Source: CAD feature listing. Evaluate the final solid. Frame: model axes, mm. A direction names the side the tool comes from. Give positions to 0.01 mm unless a question says otherwise; leave off trailing zeros. Loops run counter-clockwise (first coordinate to the right, second up) from the corner with the lowest first, then second, coordinate; pieces in that order, holes last.
Autodesk Inventor part; units mm, degrees
ref_plane "YZ Plane" through (0, 0, 0) normal (1, 0, 0) x (0, 1, 0)
ref_plane "XZ Plane" through (0, 0, 0) normal (0, 1, 0) x (-1, 0, 0)
ref_plane "XY Plane" through (0, 0, 0) normal (0, 0, 1) x (1, 0, 0)
sketch "Sketch1" plane through (0, 0, 0) normal (0, 1, 0) x (-1, 0, 0)
  line L0 (0, 0) -> (21.7678, 0)
  line L1 (21.7678, 0) -> (21.7678, -12.7)
  line L2 (21.7678, -12.7) -> (0, -12.7)
  line L3 (0, -12.7) -> (0, 0)
  circle A0 centre (25.7678, -10.95) radius 1.75
  circle A1 centre (-4, -1.75) radius 1.75
  circle A2 centre (25.7678, -10.95) radius 2.75
  circle A3 centre (-4, -1.75) radius 2.75
  line L4 (-1, -13.7) -> (22.7678, -13.7)
  line L5 (22.7678, -13.7) -> (22.7678, 1)
  line L6 (22.7678, 1) -> (-1, 1)
  line L7 (-1, 1) -> (-1, -13.7)
  line L8 (25.7678, -13.7) -> (22.7678, -13.7)
  line L9 (25.7678, -8.2) -> (22.7678, -8.2)
  line L10 (-4, 1) -> (-1, 1)
  line L11 (-4, -4.5) -> (-1, -4.5)
  dimension "d0" = 21.7678
  dimension "d1" = 12.7
  dimension "d2" = 3.5
  dimension "d3" = 3.5
  dimension "d4" = 4
  dimension "d5" = 4
  dimension "d6" = 5.5
  dimension "d7" = 5.5
extrude "Extrusion1" add sketch "Sketch1" along normal blind 2 contours L0 L1 L2 L3 | A2 | A2 L8 L5 L9 | L5 L4 L7 L6 | L7 L11 A3 L10 | A3
equation "\"d3\" = d2"
equation "\"d5\" = d4"
equation "\"d7\" = d6"
properties part number "HDMI Mount"
(1) Reachability of faces 1 (the flat face through (-22.768, 1, -4)), 2 (the flat face through (1, 1, -9)), 3 (the cylindrical face through (-24.02, 0.99, -11.03)) from +Z, -Z, +X, -X, +Y, -Y: full face, straight path, thin tool, end or side. Return the list, or none.
A:
face 1: +Z, -X, +Y, -Y
face 2: -Z, +X, +Y, -Y
face 3: +Y, -Y
(2) Section A-A, the plane y = 0.7. Return the cut outline in (x, z), then the cut area to 3 significant figures.
A:
outline: (-25.77, -13.7) - (1, -13.7) - (1, -4.5) - (4, -4.5) arc R2.75 ccw to (4, 1) - (-22.77, 1) - (-22.77, -8.2) - (-25.77, -8.2) arc R2.75 ccw to start; hole circle Ø3.5 at (-25.77, -10.95); hole circle Ø3.5 at (4, -1.75)
area: 387 mm2
(3) First-contact query: pin 1 (1 mm diameter, centred on y = 1, z = -9, fed in from -X); pin 2 (0.6 mm diameter, centred on y = 1, z = -10.5, fed in from +X). Flat tips, straight axial feed; report the tip coordinate or a pass-through.
A:
pin 1: stops at x = -28.1
pin 2: stops at x = 1
(4) Ray query, line 1 along Z through (x, y) = (4, 1.5); line 2 along X through (y, z) = (1.55, -7.5); line 3 along X through (y, z) = (1.1, -2.75). Return the intervals inside material, ascending.
A:
line 1: z = -4.5 to -3.5, 0 to 1
line 2: x = -22.77 to 1
line 3: x = -22.77 to 2.56, 5.44 to 6.56
(5) Section B-B, the plane z = -10.95. Return the cut outline in (x, y).
A:
outline: (-28.52, 0) - (-27.52, 0) - (-27.52, 2) - (-28.52, 2) - close; (-24.02, 0) - (1, 0) - (1, 2) - (-24.02, 2) - close
(6) Section C-C, the plane z = -2.25. Return the cut outline in (x, y), then the cut area to 3 significant figures.
A:
outline: (-22.77, 0) - (2.32, 0) - (2.32, 2) - (-22.77, 2) - close; (5.68, 0) - (6.7, 0) - (6.7, 2) - (5.68, 2) - close
area: 52.2 mm2
(7) Mould query, pull axis X, two halves, no side actions, for faces 4 (the cylindrical face through (-28.517, 0.986, -10.89)), 5 (the cylindrical face through (6.75, 0.99, -1.81)), 6 (the flat face through (-11, 2, -6)), 7 (the cylindrical face through (5.4, 1, -0.7)). Classes: pulls with the +X half, pulls with the -X half, needs draft (parallel to the pull), parting line crosses it, or undercut.
A:
face 4: pulls with the -X half
face 5: pulls with the +X half
face 6: needs draft
face 7: undercut
